Read the model definition and answer for the solid it produces. Units are mm, in the model's axes. A direction names the side the tool comes from. Give positions to 0.01 mm unless a question says otherwise; leave off trailing zeros. Write each loop counter-clockwise with the first axis right and the second up, starting at its lowest first coordinate (ties: lowest second). Pieces come first, ordered by that corner, then holes. Notation, with made-up numbers: M 78.5,29 L 115.5,29 A30 cw 115.5,55 Z; hole C 61.5,81.25 d8. An arc over 180 degrees is marked long. Put each result on its own line as item: value.
from build123d import *

# Parameters (mm, degrees)
CHAMFER_1_SIZE           = 1
SKETCH_8_R               = 1.5
CUT_EXTRUDE_1_DEPTH      = 30
PATTERN_CIRCULAR_1_COUNT = 4


with BuildPart() as part:
    # Эскиз7 → Повернуть1 (revolve)
    with BuildSketch(Plane(origin=(0, 0, 0), x_dir=(0, 0, -1), z_dir=(1, 0, 0)), mode=Mode.PRIVATE) as revolve_1_sk:
        Polygon((10, 0), (15, 0), (15, 12), (13.5, 12), (13.5, 13.5), (15, 13.5), (15, 30.5), (17, 30.5), (17, 32.5), (0, 32.5), (0, 2.5), (10, 2.5), align=None)
    revolve(revolve_1_sk.sketch.rotate(Axis((0, 32.703148984, 0), (0, -1, 0)), 180), axis=Axis((0, 32.703148984, 0), (0, -1, 0)))

    # Фаска1
    chamfer_1_edges = [part.edges().sort_by_distance(p)[0] for p in [
        (0, 0, -15),
    ]]
    chamfer(chamfer_1_edges, length=CHAMFER_1_SIZE)

    # Эскиз8 → Вырез-Вытянуть1 (cut)
    with BuildSketch(Plane.XZ.offset(-2.5)):
        with Locations(Location((7, 0, 0), (0, 0, 270))):
            Circle(SKETCH_8_R)
    cut_extrude_1 = extrude(amount=-CUT_EXTRUDE_1_DEPTH, mode=Mode.SUBTRACT)

    # Круговой массив1: Вырез-Вытянуть1 ×4 about axis
    pattern_circular_1_axis = Axis((0, 0, 0), (0, 1, 0))
    for i in range(1, PATTERN_CIRCULAR_1_COUNT):
        add(cut_extrude_1.rotate(pattern_circular_1_axis, i * 360 / PATTERN_CIRCULAR_1_COUNT), mode=Mode.SUBTRACT)


solid = part.part
(1) Section C-C on y = 28 is taken. Determine the outline of the cut face in (x, z).
Result:
outline: C 0,0 d30; hole C -7,0 d3; hole C 0,-7 d3; hole C 0,7 d3; hole C 7,0 d3
(2) Section D-D on y = 2 is taken. Determine the outline of the cut face in (x, z), and give its area (3 significant figures).
Result:
outline: C 0,0 d30; hole C 0,0 d20
area: 393 mm²
(3) Straight lines are drawn through the part: line 1 along X through (y, z) = (9.25, 0); line 2 along Y through (x, z) = (-3.5, 8); line 3 along X through (y, z) = (11.5, -8). For each, find the intervals that lie inside material, in ascending order. Write a range as from..to.
Result:
line 1: x = -15..-8.5, -5.5..5.5, 8.5..15
line 2: y = 2.5..32.5
line 3: x = -12.69..-1.12, 1.12..12.69
(4) For a pull along Z with two mould halves and no side action, classify faces 4 (the face through (-5.536, 17.29, -0.325)), 5 (the face through (13.18, 12.76, -2.93)), 6 (the face through (-7.85, 13.5, 11.18)), 7 (the face through (0, 2.5, 0)) as +Z half, -Z half, draft (parallel to the pull), parting line (faces both ways), or undercut.
Result:
face 4: undercut
face 5: parting line
face 6: draft
face 7: undercut
(5) Given pin 1 Ø2 at (x, y) = (-3.5, 17.5) entering from +Z; pin 2 Ø2.5 at (x, z) = (7, 0) entering from -Y; pin 3 Ø1 at (x, y) = (-11.5, 26) entering from +Z; pin 4 Ø5 at (y, z) = (6.5, -11) entering from -X, each flat-ended and moving along its own axis, determine where each tip first touches the part or whether it passes through.
Result:
pin 1: stops at z = 14.79
pin 2: passes through
pin 3: stops at z = 10.2
pin 4: stops at x = -12.36
(6) Section A-A on z = 0 is taken. Give the number of separate pieces and of enclosed holes in the cut face, and give its area (4 significant figures).
Result:
separate pieces: 3
enclosed holes: 0
area: 747.5 mm²
(7) Which of the six approach directions +Z, -Z, +X, -X, +Y, -Y give full straight-line access (tool end or side, diameter ignored) to faces 1 (the face through (-7.85, 12, -11.18)), 2 (the face through (0, 1, -10)), 3 (the face through (-16.855, 31.514, -2.213))?
Result:
face 1: none
face 2: -Y
face 3: +Y, -Y
